from build123d import *

# Parameters (mm, degrees)
F0_W          = 3.0335542979
F0_H          = 151.8673300743
F1_DEPTH      = 19.05
F1_DEPTH_BACK = 19.05
F2_ANGLE      = 9.5
F3_W          = 37.5402383506
F3_H          = 2.8439536691
F4_DEPTH      = 50.8
F5_W          = 36.9333513081
F5_H          = 2.0887702703
F6_DEPTH      = 19.05
F6_DEPTH_BACK = 19.05
F7_W          = 2.0887777209
F7_H          = 4.9371048808
F8_DEPTH      = 19.05
F8_DEPTH_BACK = 19.05
F9_W          = 37.9011612386
F9_H          = 4.8097893596
F10_DEPTH     = 2.1336


with BuildPart() as f1:
    # F0 (on Right) → F1 (new body, two sides)
    with BuildSketch(Plane.YZ) as f1_sk:
        with Locations((-0.0947989174, 0)):
            Rectangle(F0_W, F0_H)
    extrude(amount=F1_DEPTH)
    extrude(f1_sk.sketch, amount=-F1_DEPTH_BACK)


with BuildPart() as f1_1:
    # F2: moved
    add(f1.part.rotate(Axis((0, -1.6115760664, -75.9336650372), (-1, 0, 0)), F2_ANGLE))

    # F3 (on Front) → F4 (join)
    with BuildSketch(Plane.XZ):
        with Locations((-0.0947974622, -74.3220858276)):
            Rectangle(F3_W, F3_H)
    extrude(amount=-F4_DEPTH)

    # F5 (on Right) → F6 (join, two sides)
    with BuildSketch(Plane.YZ) as f6_sk:
        with Locations((18.4666756541, 74.3191987276)):
            Rectangle(F5_W, F5_H)
    extrude(amount=F6_DEPTH)
    extrude(f6_sk.sketch, amount=-F6_DEPTH_BACK)

    # F7 (on Right) → F8 (join, two sides)
    with BuildSketch(Plane.YZ) as f8_sk:
        with Locations((36.07885167, 75.7433660328)):
            Rectangle(F7_W, F7_H)
    extrude(amount=F8_DEPTH)
    extrude(f8_sk.sketch, amount=-F8_DEPTH_BACK)

    # F9 (on Front) → F10 (join)
    with BuildSketch(Plane.XZ):
        with Locations((-0.1923916861, 75.5367614329)):
            Rectangle(F9_W, F9_H)
    extrude(amount=-F10_DEPTH)


solid = f1_1.part
Geometry check sheet. Reference: the model listing, model coordinates, mm. A direction names the side the tool comes from. Round coordinates to 2 decimals unless told otherwise and drop trailing zeros. Loops run counter-clockwise (first coordinate to the right, second up) from the corner with the lowest first, then second, coordinate; pieces in that order, holes last.
Item 1: Cross-section at B-B on x = -9. Record the boundary of the cut face in (y, z).
Item 2: Cross-section at D-D on z = 67. Record the boundary of the cut face in (x, y).
Item 3: Access from +Z, -Z, +X, -X, +Y, -Y to the whole of each face (thin tool, end or side, straight path). Record for faces 4 (the flat face through (-18.865, 26, -74)), 5 (the flat face through (0, 35.034, 77)), 6 (the flat face through (0, 37.123, 76)), 7 (the flat face through (18.675, 26, -74)).
Item 4: Mould release check, pull along Y, two halves, no side actions. Record for faces 1 (the flat face through (0, 50.8, -74)), 2 (the flat face through (19.05, 13, 1)), 3 (the flat face through (0, 17, 75.364)): pulls with the +Y half, pulls with the -Y half, needs draft (parallel to the pull), parting line crosses it, or undercut.
Item 5: Cross-section at A-A on y = 5.5. Record the boundary of the cut face in (x, z), then the cut area to 3 significant figures.
Item 6: Gauge pin test, flat ends, axial feed: pin 1 (2.5 mm diameter, centred on y = 1, z = 77, fed in from +X); pin 2 (1.4 mm diameter, centred on x = 9, z = 74.5, fed in from +Y); pin 3 (12 mm diameter, centred on x = 2, y = 10.5, fed in from +Z). Record the tip position at first contact, or that the pin passes through.
Item 7: Thickness scan on line 1 (Z direction, x = 12, y = 27); line 2 (Z direction, x = -16.5, y = 39.5); line 3 (X direction, y = 16, z = 23). Record the ranges inside material, lowest first.
Item 8: Cross-section at C-C on y = 47. Record the boundary of the cut face in (x, z).
Answer sheet:
1. outline: (-1.61, -75.93) - (1.38, -76.43) - (1.5, -75.74) - (50.8, -75.74) - (50.8, -72.9) - (1.97, -72.9) - (26.43, 73.27) - (37.12, 73.27) - (37.12, 78.21) - (35.03, 78.21) - (35.03, 75.36) - (2.13, 75.36) - (2.13, 77.94) - (0, 77.94) - (0, 73.13) - (2.13, 73.13) - (2.13, 73.27) - (23.36, 73.27) - close
2. outline: (-19.05, 22.31) - (19.05, 22.31) - (19.05, 25.38) - (-19.05, 25.38) - close
3. face 4: -Z, -X, +Y
3. face 5: +Z, +X, -X
3. face 6: +Z, +X, -X, +Y
3. face 7: -Z, +X, +Y
4. face 1: pulls with the +Y half
4. face 2: needs draft
4. face 3: undercut
5. outline: (-19.05, -51.82) - (19.05, -51.82) - (19.05, -33.44) - (-19.05, -33.44) - close; (-19.05, 73.27) - (19.05, 73.27) - (19.05, 75.36) - (-19.05, 75.36) - close; (-18.86, -75.74) - (18.68, -75.74) - (18.68, -72.9) - (-18.86, -72.9) - close
5. area: 887 mm2
6. pin 1: stops at x = 18.76
6. pin 2: stops at y = 37.12
6. pin 3: stops at z = 75.36
7. line 1: z = -75.74 to -72.9, 73.27 to 75.36
7. line 2: z = -75.74 to -72.9
7. line 3: x = -19.05 to 19.05
8. outline: (-18.86, -75.74) - (18.68, -75.74) - (18.68, -72.9) - (-18.86, -72.9) - close
